Geometry check sheet. Reference: the model listing, model coordinates, mm. A direction names the side the tool comes from. Round coordinates to 2 decimals unless told otherwise and drop trailing zeros. Order: outer loops, then holes, each group sorted by start corner. A loop starts at its lowest first (then second) coordinate and runs counter-clockwise, first axis right, second up. Notation, with made-up numbers: (18, -7.5) - (25, -7.5) arc R17 cw to (25, 16.5) - close; hole circle Ø1 at (-14.5, 81.5). An arc over 180 degrees is marked (long way). Return JSON: item names as keys, results as strings. Group by question number.
Q1. Sectioned sample at B-B, the plane x = 0. Record the cut outline in (y, z), then the cut area to 3 significant figures.
Q2. Sectioned sample at A-A, the plane z = 8.4. Record the cut outline in (x, y).
Q3. Gauge pin test, flat ends, axial feed: pin 1 Ø2.5 at (x, z) = (-0.5, 17) entering from +Y; pin 2 Ø4.5 at (x, y) = (4.5, 12.5) entering from -Z; pin 3 Ø12 at (x, z) = (-6, -13) entering from +Y; pin 4 Ø2.5 at (x, z) = (0, -14.5) entering from -Y. Record the tip position at first contact, or that the pin passes through.
Q4. Draft check along X on faces 6 (the flat face through (-10, 4.6, 4.2)), 7 (the flat face through (0, 5, -3)), 8 (the flat face through (0, 16.37, 16)). Enter one of: pulls with the +X half, pulls with the -X half, needs draft (parallel to the pull), parting line crosses it, or undercut.
Q5. Tool access check on faces 1 (the flat face through (0, 12, 13.5)), 2 (the flat face through (-5.255, 19, 16)), 3 (the cylindrical face through (7.5, 15.5, 15.2)), 4 (the flat face through (0, 2, -18.5)), 5 (the cylindrical face through (0.51, 2.54, -12.88)). Record the directions out of +Z, -Z, +X, -X, +Y, -Y that give a thin tool (end or side, any length) a straight path to the whole face; none if there is none.
Q6. Sectioned sample at C-C, the plane z = 14.5. Record the cut outline in (x, y) (3 decimals), then the cut area to 3 significant figures.
Q7. Sectioned sample at D-D, the plane y = 13.75. Record the cut outline in (x, z).
Q8. Material ranges on line 1 along X through (y, z) = (15, 16); line 2 along X through (y, z) = (17, 16) (3 decimals); line 3 along X through (y, z) = (3, -14.5), recorded low to high.
```python
from build123d import *

# Parameters (mm, degrees)
SKETCH2_W                  = 20
SKETCH2_H                  = 37
EXTRUDE1_DEPTH             = 5
F_3_4_3_4_DIAMETER_HOLE1_D = 3.4
LPATTERN1_COUNT            = 2
LPATTERN1_PITCH            = 22.9
SKETCH5_W                  = 20
SKETCH5_H                  = 5
EXTRUDE2_DEPTH             = 14.5
LPATTERN2_COUNT            = 2
LPATTERN2_PITCH            = 15
SKETCH6_W                  = 10.51
SKETCH6_H                  = 5
EXTRUDE3_DEPTH             = 1.5
SKETCH7_W                  = 6.51
SKETCH7_H                  = 5
EXTRUDE4_DEPTH             = 1.63


with BuildPart() as part:
    # Sketch2 → Extrude1 (new body)
    with BuildSketch(Plane(origin=(0, 0, 0), x_dir=(1, 0, 0), z_dir=(0, 1, 0))):
        Rectangle(SKETCH2_W, SKETCH2_H)
    extrude(amount=EXTRUDE1_DEPTH)

    # Ø3.4 (3.4) Diameter Hole1 (through all)
    with Locations(Plane(origin=(0, 0, -14.5), x_dir=(0, 0, -1), z_dir=(0, -1, 0))):
        with Locations((0, 0)):
            f_3_4_3_4_diameter_hole1 = Hole(F_3_4_3_4_DIAMETER_HOLE1_D / 2)

    # LPattern1: Ø3.4 (3.4) Diameter Hole1 ×2
    with Locations(*[(0, 0, i * LPATTERN1_PITCH) for i in range(1, LPATTERN1_COUNT)]):
        add(f_3_4_3_4_diameter_hole1, mode=Mode.SUBTRACT)

    # Sketch5 → Extrude2 (add)
    with BuildSketch(Plane(origin=(0, 5, 0), x_dir=(1, 0, 0), z_dir=(0, 1, 0))):
        with Locations((0, -16)):
            Rectangle(SKETCH5_W, SKETCH5_H)
    extrude(amount=EXTRUDE2_DEPTH)

    # Sketch10 → M2x0.4 Tapped Hole1 (revolve, cut)
    with BuildSketch(Plane(origin=(-7.5, 19.5, 16), x_dir=(0, 0, 1), z_dir=(1, 0, 0))):
        Polygon((0, 0), (0, 8.680688495), (0.8, 8.2), (0.8, 0), align=None)
    m2x0_4_tapped_hole1 = revolve(axis=Axis((-7.5, 25.85, 16), (0, -1, 0)), mode=Mode.SUBTRACT)

    # LPattern2: M2x0.4 Tapped Hole1 ×2
    with Locations(*[(i * LPATTERN2_PITCH, 0, 0) for i in range(1, LPATTERN2_COUNT)]):
        add(m2x0_4_tapped_hole1, mode=Mode.SUBTRACT)

    # Sketch6 → Extrude3 (cut)
    with BuildSketch(Plane(origin=(0, 19.5, 0), x_dir=(-1, 0, 0), z_dir=(0, 1, 0))):
        with Locations((0, 16)):
            Rectangle(SKETCH6_W, SKETCH6_H)
    extrude(amount=-EXTRUDE3_DEPTH, mode=Mode.SUBTRACT)

    # Sketch7 → Extrude4 (cut)
    with BuildSketch(Plane(origin=(0, 18, 0), x_dir=(-1, 0, 0), z_dir=(0, 1, 0))):
        with Locations((0, 16)):
            Rectangle(SKETCH7_W, SKETCH7_H)
    extrude(amount=-EXTRUDE4_DEPTH, mode=Mode.SUBTRACT)


solid = part.part
```
Reply:
{
 "1": {"outline": "(0, -18.5) - (5, -18.5) - (5, -16.2) - (0, -16.2) - close; (0, -12.8) - (5, -12.8) - (5, 6.7) - (0, 6.7) - close; (0, 10.1) - (5, 10.1) - (5, 13.5) - (16.37, 13.5) - (16.37, 18.5) - (0, 18.5) - close", "area": "208 mm^2"},
 "2": {"outline": "(-10, 0) - (-1.7, 0) - (-1.7, 5) - (-10, 5) - close; (1.7, 0) - (10, 0) - (10, 5) - (1.7, 5) - close"},
 "3": {"pin 1": "y = 16.37", "pin 2": "z = 13.5", "pin 3": "y = 5", "pin 4": "through"},
 "4": {"face 6": "pulls with the -X half", "face 7": "needs draft", "face 8": "undercut"},
 "5": {"face 1": "-Z, +X, -X, +Y", "face 2": "+Z, -Z, +Y", "face 3": "+Y", "face 4": "-Z, +X, -X, +Y, -Y", "face 5": "+Y, -Y"},
 "6": {"outline": "(-10, 0) - (10, 0) - (10, 19.5) - (5.255, 19.5) - (5.255, 18) - (3.255, 18) - (3.255, 16.37) - (-3.255, 16.37) - (-3.255, 18) - (-5.255, 18) - (-5.255, 19.5) - (-10, 19.5) - close", "area": "364 mm^2"},
 "7": {"outline": "(-10, 13.5) - (10, 13.5) - (10, 18.5) - (-10, 18.5) - close; hole circle Ø1.6 at (-7.5, 16); hole circle Ø1.6 at (7.5, 16)"},
 "8": {"line 1": "-10 to -8.3, -6.7 to 6.7, 8.3 to 10", "line 2": "-10 to -8.3, -6.7 to -3.255, 3.255 to 6.7, 8.3 to 10", "line 3": "-10 to -1.7, 1.7 to 10"}
}
